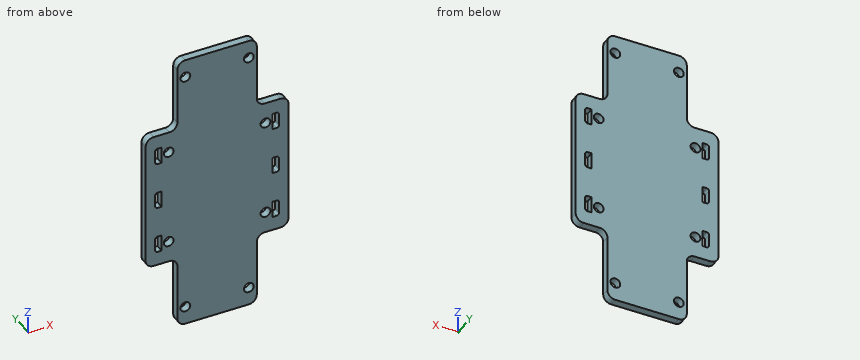
from build123d import *

# Parameters (mm, degrees)
BOSS_EXTRUDE1_DEPTH = 2.5
SKETCH2_R           = 1.55
CUT_EXTRUDE1_DEPTH  = 51.373604199
CUT_EXTRUDE2_DEPTH  = 51.373604199
FILLET2_R           = 2.5
FILLET3_R           = 2.5


with BuildPart() as part:
    # Sketch1 → Boss-Extrude1 (new body)
    with BuildSketch(Plane(origin=(0, 0, 0), x_dir=(1, 0, 0), z_dir=(0, 1, 0))):
        Polygon((12.5, -45), (-12.5, -45), (-12.5, -22), (-22.5, -22), (-22.5, 22), (-12.5, 22), (-12.5, 45), (12.5, 45), (12.5, 22), (22.5, 22), (22.5, -22), (12.5, -22), align=None)
    extrude(amount=BOSS_EXTRUDE1_DEPTH)

    # Sketch2 → Cut-Extrude1 (cut, through all)
    with BuildSketch(Plane(origin=(0, 2.5, 0), x_dir=(1, 0, 0), z_dir=(0, 1, 0))):
        with Locations(Location((-15.25, 15.25, 0), (0, 0, 270))):
            Circle(SKETCH2_R)
        with Locations(Location((15.25, 15.25, 0), (0, 0, 270))):
            Circle(SKETCH2_R)
        with Locations(Location((15.25, -15.25, 0), (0, 0, 90))):
            Circle(SKETCH2_R)
        with Locations(Location((-15.25, -15.25, 0), (0, 0, 90))):
            Circle(SKETCH2_R)
        with Locations(Location((-10, 39.25, 0), (0, 0, 270))):
            Circle(SKETCH2_R)
        with Locations(Location((-10, -39.25, 0), (0, 0, 90))):
            Circle(SKETCH2_R)
        with Locations(Location((10, -39.25, 0), (0, 0, 270))):
            Circle(SKETCH2_R)
        with Locations(Location((10, 39.25, 0), (0, 0, 90))):
            Circle(SKETCH2_R)
    extrude(amount=-CUT_EXTRUDE1_DEPTH, mode=Mode.SUBTRACT)

    # Sketch3 → Cut-Extrude2 (cut, through all)
    with BuildSketch(Plane(origin=(0, 2.5, 0), x_dir=(1, 0, 0), z_dir=(0, 1, 0))):
        with BuildLine():
            Line((-17.5, -2.6), (-18.75, -2.6))
            ThreePointArc((-18.75, -2.6), (-19.280330086, -2.380330086), (-19.5, -1.85))
            Line((-19.5, -1.85), (-19.5, 1.85))
            ThreePointArc((-19.5, 1.85), (-19.280330086, 2.380330086), (-18.75, 2.6))
            Line((-18.75, 2.6), (-17.5, 2.6))
            Line((-17.5, 2.6), (-17.5, -2.6))
        make_face()
        with BuildLine():
            Line((-17.5, 12.4), (-18.75, 12.4))
            ThreePointArc((-18.75, 12.4), (-19.280330086, 12.619669914), (-19.5, 13.15))
            Line((-19.5, 13.15), (-19.5, 16.85))
            ThreePointArc((-19.5, 16.85), (-19.280330086, 17.380330086), (-18.75, 17.6))
            Line((-18.75, 17.6), (-17.5, 17.6))
            Line((-17.5, 17.6), (-17.5, 12.4))
        make_face()
        with BuildLine():
            Line((-17.5, 27.4), (-18.75, 27.4))
            ThreePointArc((-18.75, 27.4), (-19.280330086, 27.619669914), (-19.5, 28.15))
            Line((-19.5, 28.15), (-19.5, 31.85))
            ThreePointArc((-19.5, 31.85), (-19.280330086, 32.380330086), (-18.75, 32.6))
            Line((-18.75, 32.6), (-17.5, 32.6))
            Line((-17.5, 32.6), (-17.5, 27.4))
        make_face()
        with BuildLine():
            Line((19.5, 28.15), (19.5, 31.85))
            ThreePointArc((19.5, 31.85), (19.280330086, 32.380330086), (18.75, 32.6))
            Line((18.75, 32.6), (17.5, 32.6))
            Line((17.5, 32.6), (17.5, 27.4))
            Line((17.5, 27.4), (18.75, 27.4))
            ThreePointArc((18.75, 27.4), (19.280330086, 27.619669914), (19.5, 28.15))
        make_face()
        with BuildLine():
            Line((19.5, 13.15), (19.5, 16.85))
            ThreePointArc((19.5, 16.85), (19.280330086, 17.380330086), (18.75, 17.6))
            Line((18.75, 17.6), (17.5, 17.6))
            Line((17.5, 17.6), (17.5, 12.4))
            Line((17.5, 12.4), (18.75, 12.4))
            ThreePointArc((18.75, 12.4), (19.280330086, 12.619669914), (19.5, 13.15))
        make_face()
        with BuildLine():
            Line((19.5, -1.85), (19.5, 1.85))
            ThreePointArc((19.5, 1.85), (19.280330086, 2.380330086), (18.75, 2.6))
            Line((18.75, 2.6), (17.5, 2.6))
            Line((17.5, 2.6), (17.5, -2.6))
            Line((17.5, -2.6), (18.75, -2.6))
            ThreePointArc((18.75, -2.6), (19.280330086, -2.380330086), (19.5, -1.85))
        make_face()
        with BuildLine():
            Line((17.5, -12.4), (18.75, -12.4))
            ThreePointArc((18.75, -12.4), (19.280330086, -12.619669914), (19.5, -13.15))
            Line((19.5, -13.15), (19.5, -16.85))
            ThreePointArc((19.5, -16.85), (19.280330086, -17.380330086), (18.75, -17.6))
            Line((18.75, -17.6), (17.5, -17.6))
            Line((17.5, -17.6), (17.5, -12.4))
        make_face()
        with BuildLine():
            Line((17.5, -27.4), (18.75, -27.4))
            ThreePointArc((18.75, -27.4), (19.280330086, -27.619669914), (19.5, -28.15))
            Line((19.5, -28.15), (19.5, -31.85))
            ThreePointArc((19.5, -31.85), (19.280330086, -32.380330086), (18.75, -32.6))
            Line((18.75, -32.6), (17.5, -32.6))
            Line((17.5, -32.6), (17.5, -27.4))
        make_face()
        with BuildLine():
            Line((-19.5, -28.15), (-19.5, -31.85))
            ThreePointArc((-19.5, -31.85), (-19.280330086, -32.380330086), (-18.75, -32.6))
            Line((-18.75, -32.6), (-17.5, -32.6))
            Line((-17.5, -32.6), (-17.5, -27.4))
            Line((-17.5, -27.4), (-18.75, -27.4))
            ThreePointArc((-18.75, -27.4), (-19.280330086, -27.619669914), (-19.5, -28.15))
        make_face()
        with BuildLine():
            Line((-19.5, -13.15), (-19.5, -16.85))
            ThreePointArc((-19.5, -16.85), (-19.280330086, -17.380330086), (-18.75, -17.6))
            Line((-18.75, -17.6), (-17.5, -17.6))
            Line((-17.5, -17.6), (-17.5, -12.4))
            Line((-17.5, -12.4), (-18.75, -12.4))
            ThreePointArc((-18.75, -12.4), (-19.280330086, -12.619669914), (-19.5, -13.15))
        make_face()
    extrude(amount=-CUT_EXTRUDE2_DEPTH, mode=Mode.SUBTRACT)

    # Fillet2
    fillet2_edges = [part.edges().sort_by_distance(p)[0] for p in [
        (-12.5, 1.25, 22),
        (-22.5, 1.25, 22),
        (-22.5, 1.25, -22),
        (-12.5, 1.25, -22),
        (12.5, 1.25, -22),
        (22.5, 1.25, -22),
        (22.5, 1.25, 22),
        (12.5, 1.25, 22),
    ]]
    fillet(fillet2_edges, radius=FILLET2_R)

    # Fillet3
    fillet3_edges = [part.edges().sort_by_distance(p)[0] for p in [
        (12.5, 1.25, 45),
        (-12.5, 1.25, 45),
        (-12.5, 1.25, -45),
        (12.5, 1.25, -45),
    ]]
    fillet(fillet3_edges, radius=FILLET3_R)


solid = part.part
Part model, mm, in its own coordinate system. Give positions to 0.01 mm unless a question says otherwise; leave off trailing zeros. Loops run counter-clockwise (first coordinate to the right, second up) from the corner with the lowest first, then second, coordinate; pieces in that order, holes last.
(1) Pin check, flat tips, straight feed: pin 1 (1.2 mm diameter, centred on y = 2, z = -36, fed in from -X); pin 2 (0.6 mm diameter, centred on x = 18, y = 1, fed in from +Z); pin 3 (1.4 mm diameter, centred on x = 18, y = 1, fed in from -Z). Stop position of each tip, or through.
Return value:
pin 1: stops at x = -12.5
pin 2: stops at z = 22
pin 3: stops at z = -22
(2) Band-saw the part on C-C (y = 1). Count the separate pieces of the cut face and the enclosed holes in it, and give its area (3 significant figures).
Return value:
separate pieces: 1
enclosed holes: 14
area: 3,000 mm2
(3) Band-saw the part on A-A (z = 15.25). Write the cut outline in (x, y).
Return value:
outline: (-22.5, 0) - (-19.5, 0) - (-19.5, 2.5) - (-22.5, 2.5) - close; (-17.5, 0) - (-16.8, 0) - (-16.8, 2.5) - (-17.5, 2.5) - close; (-13.7, 0) - (13.7, 0) - (13.7, 2.5) - (-13.7, 2.5) - close; (16.8, 0) - (17.5, 0) - (17.5, 2.5) - (16.8, 2.5) - close; (19.5, 0) - (22.5, 0) - (22.5, 2.5) - (19.5, 2.5) - close
(4) Drill centre lines: line 1 along X through (y, z) = (0.3, 2); line 2 along X through (y, z) = (1.25, -39.25); line 3 along X through (y, z) = (0.4, -15.5). Where is each one in solid material? Low to high.
Return value:
line 1: x = -22.5 to -19.48, -17.5 to 17.5, 19.48 to 22.5
line 2: x = -12.5 to -11.55, -8.45 to 8.45, 11.55 to 12.5
line 3: x = -22.5 to -19.5, -17.5 to -16.78, -13.72 to 13.72, 16.78 to 17.5, 19.5 to 22.5
(5) Band-saw the part on D-D (z = -28). Write the cut outline in (x, y).
Return value:
outline: (-12.5, 0) - (12.5, 0) - (12.5, 2.5) - (-12.5, 2.5) - close
(6) Band-saw the part on B-B (z = 39.25). Write the cut outline in (x, y).
Return value:
outline: (-12.5, 0) - (-11.55, 0) - (-11.55, 2.5) - (-12.5, 2.5) - close; (-8.45, 0) - (8.45, 0) - (8.45, 2.5) - (-8.45, 2.5) - close; (11.55, 0) - (12.5, 0) - (12.5, 2.5) - (11.55, 2.5) - close
